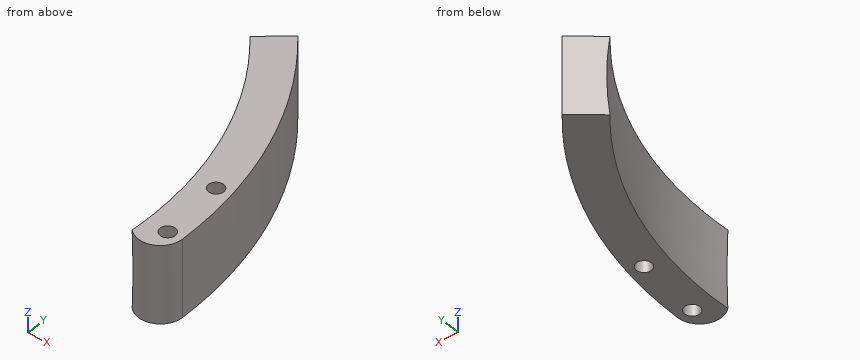
```python
from build123d import *

# Parameters (mm, degrees)
BOSS_EXTRUDE1_DEPTH      = 16.66875
BOSS_EXTRUDE1_DEPTH_BACK = 16.66875
SKETCH2_R                = 3.2639


with BuildPart() as part:
    # Sketch2 → Boss-Extrude1 (new, two sides: drawn at the far end of the back side and taken through both)
    with BuildSketch(Plane.XY.offset(-BOSS_EXTRUDE1_DEPTH_BACK)):
        with BuildLine():
            Line((116.745173131, 97.960831716), (131.338319773, 110.205935681))
            ThreePointArc((131.338319773, 110.205935681), (161.110299834, 58.639353573), (171.45, 0))
            ThreePointArc((171.45, 0), (161.925, -9.525), (152.4, 0))
            ThreePointArc((152.4, 0), (143.209155408, 52.123869843), (116.745173131, 97.960831716))
        make_face()
        with Locations((165.1, 0)):
            Circle(SKETCH2_R, mode=Mode.SUBTRACT)
        with Locations((162.591760022, 28.669314133)):
            Circle(SKETCH2_R, mode=Mode.SUBTRACT)
    extrude(amount=BOSS_EXTRUDE1_DEPTH + BOSS_EXTRUDE1_DEPTH_BACK)

    # Sketch3 → Cut-Revolve2 (revolve, cut)
    with BuildSketch(Plane(origin=(0, 0, 0), x_dir=(1, 0, 0), z_dir=(0, 1, 0))):
        with BuildLine():
            Line((31.75, 0), (31.75, 124.757705173))
            ThreePointArc((31.75, 124.757705173), (156.507705173, 0), (31.75, -124.757705173))
            Line((31.75, -124.757705173), (31.75, 0))
        make_face()
    revolve(axis=Axis((0, 0, 1000), (0, 0, -1)), mode=Mode.SUBTRACT)


solid = part.part
```
Geometry check sheet. Reference: the model listing, model coordinates, mm. Give positions to 0.01 mm unless a question says otherwise; leave off trailing zeros.
1) Section check A-A, the plane z = 5. State how many separate pieces and enclosed holes the cut face has, and give its area (3 significant figures).
2) Material ranges on L1, parallel to X at y = 26.5, z = -11; L2, parallel to X at y = 45.5, z = -7; L3, parallel to X at y = -3, z = 4.5, recorded low to high.
3) Gauge pin test, flat ends, axial feed: pin 1 (2 mm diameter, centred on x = 140.5, z = -0.5, fed in from +Y); pin 2 (4 mm diameter, centred on y = 52, z = 12.5, fed in from +X); pin 3 (5 mm diameter, centred on x = 165.1, y = 0, fed in from +Z); pin 4 (1.5 mm diameter, centred on x = 136, z = -2, fed in from +Y). Record the tip position at first contact, or that the pin passes through.
Computed:
1. separate pieces: 1
1. enclosed holes: 2
1. area: 1,780 mm2
2. L1: x = 153.75 to 160.15, 165.03 to 169.39
2. L2: x = 149.54 to 165.3
2. L3: x = 156.4 to 163.81, 166.39 to 170.97
3. pin 1: stops at y = 99.67
3. pin 2: stops at x = 164
3. pin 3: passes through
3. pin 4: stops at y = 105.37
